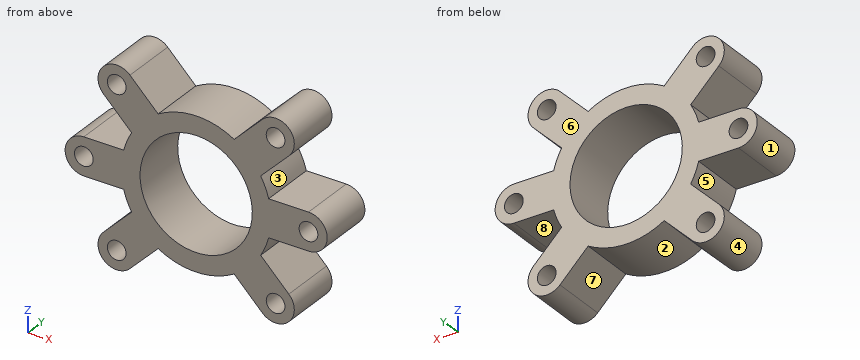
```python
from build123d import *

# Parameters (mm, degrees)
SKETCH2_R           = 30
SKETCH2_R_2         = 5
BOSS_EXTRUDE1_DEPTH = 15


with BuildPart() as part:
    # Sketch2 → Boss-Extrude1 (new, symmetric)
    with BuildSketch(Plane(origin=(0, 0, 0), x_dir=(1, 0, 0), z_dir=(0, 1, 0))):
        with BuildLine():
            Line((38.729833462, 10), (60, 10))
            ThreePointArc((60, 10), (70, 0), (60, -10))
            Line((60, -10), (38.729833462, -10))
            ThreePointArc((38.729833462, -10), (36.9551813, -15.307337295), (34.457195687, -20.315060063))
            Line((34.457195687, -20.315060063), (49.497474683, -35.355339059))
            ThreePointArc((49.497474683, -35.355339059), (49.497474683, -49.497474683), (35.355339059, -49.497474683))
            Line((35.355339059, -49.497474683), (20.315060063, -34.457195687))
            ThreePointArc((20.315060063, -34.457195687), (0, -40), (-20.315060063, -34.457195687))
            Line((-20.315060063, -34.457195687), (-35.355339059, -49.497474683))
            ThreePointArc((-35.355339059, -49.497474683), (-49.497474683, -49.497474683), (-49.497474683, -35.355339059))
            Line((-49.497474683, -35.355339059), (-34.457195687, -20.315060063))
            ThreePointArc((-34.457195687, -20.315060063), (-36.9551813, -15.307337295), (-38.729833462, -10))
            Line((-38.729833462, -10), (-60, -10))
            ThreePointArc((-60, -10), (-70, 0), (-60, 10))
            Line((-60, 10), (-38.729833462, 10))
            ThreePointArc((-38.729833462, 10), (-36.9551813, 15.307337295), (-34.457195687, 20.315060063))
            Line((-34.457195687, 20.315060063), (-49.497474683, 35.355339059))
            ThreePointArc((-49.497474683, 35.355339059), (-49.497474683, 49.497474683), (-35.355339059, 49.497474683))
            Line((-35.355339059, 49.497474683), (-20.315060063, 34.457195687))
            ThreePointArc((-20.315060063, 34.457195687), (0, 40), (20.315060063, 34.457195687))
            Line((20.315060063, 34.457195687), (35.355339059, 49.497474683))
            ThreePointArc((35.355339059, 49.497474683), (49.497474683, 49.497474683), (49.497474683, 35.355339059))
            Line((49.497474683, 35.355339059), (34.457195687, 20.315060063))
            ThreePointArc((34.457195687, 20.315060063), (36.9551813, 15.307337295), (38.729833462, 10))
        make_face()
        with Locations(Location((0, 0, 0), (0, 0, 270))):
            Circle(SKETCH2_R, mode=Mode.SUBTRACT)
        with Locations(Location((60, 0, 0), (0, 0, 270))):
            Circle(SKETCH2_R_2, mode=Mode.SUBTRACT)
        with Locations(Location((42.426406871, -42.426406871, 0), (0, 0, 270))):
            Circle(SKETCH2_R_2, mode=Mode.SUBTRACT)
        with Locations(Location((-42.426406871, -42.426406871, 0), (0, 0, 270))):
            Circle(SKETCH2_R_2, mode=Mode.SUBTRACT)
        with Locations(Location((-60, 0, 0), (0, 0, 270))):
            Circle(SKETCH2_R_2, mode=Mode.SUBTRACT)
        with Locations(Location((-42.426406871, 42.426406871, 0), (0, 0, 270))):
            Circle(SKETCH2_R_2, mode=Mode.SUBTRACT)
        with Locations(Location((42.426406871, 42.426406871, 0), (0, 0, 270))):
            Circle(SKETCH2_R_2, mode=Mode.SUBTRACT)
    extrude(amount=BOSS_EXTRUDE1_DEPTH, both=True)


solid = part.part
```
Check sheet for the modelled part. Datum: model origin and axes. Units: mm. Face numbers are marked on the shaded views. A direction names the side the tool comes from. Round coordinates to 2 decimals unless told otherwise and drop trailing zeros. Loops run counter-clockwise (first coordinate to the right, second up) from the corner with the lowest first, then second, coordinate; pieces in that order, holes last. Notation, with made-up numbers: (28, 50.5) - (49, 50.5) arc R24 ccw to (49, 80.5) - close; hole circle Ø6 at (70, 71). An arc over 180 degrees is marked (long way). Answer as a JSON object with one key per item and string values. Group by question number.
Q1. Sectioned sample at D-D, the plane x = -14.5. Enter the section's corners in (y, z), plus the area to 3 significant figures.
Q2. Set-up check for the marked faces 5, 6, 7 and 8: record each of +Z, -Z, +X, -X, +Y, -Y from which the full face is reachable in a straight line by a thin tool's end or side.
Q3. Mould release check, pull along X, two halves, no side actions. Record for the marked faces 1, 2, 3 and 4: released by +X, released by -X, zero draft, split by the parting line, or undercut.
Q4. Sectioned sample at A-A, the plane z = 0. Enter the section's corners in (x, y).
Q5. Sectioned sample at C-C, the plane y = 5. Count the separate pieces of the cut face and the enclosed holes in it, plus the area to 3 significant figures.
Q6. Gauge pin test, flat ends, axial feed: P1, Ø10.5, axis at x = -50, y = 0.5, coming from the +Z side; P2, Ø5, axis at x = -50.5, y = -9, coming from the -Z side; P3, Ø4, axis at x = 20, y = 8.5, coming from the -Z side. Record the tip position at first contact, or that the pin passes through.
Q7. Scan lines: line 1 along X through (y, z) = (0.5, 0); line 2 along Z through (x, y) = (42.5, 1.75); line 3 along Z through (x, y) = (40, 5). Record each from-to range of solid material in increasing order. Write a range as [from, to].
Q8. Sectioned sample at B-B, the plane x = 0. Enter the section's corners in (y, z), plus the area to 3 significant figures.
Solution:
{
 "1": {"outline": "(-15, -37.28) - (15, -37.28) - (15, -26.26) - (-15, -26.26) - close; (-15, 26.26) - (15, 26.26) - (15, 37.28) - (-15, 37.28) - close", "area": "661 mm²"},
 "2": {"face 5": "-X, +Y, -Y", "face 6": "+Z, -Z, +X, -X, +Y", "face 7": "-Z, +Y, -Y", "face 8": "+X, +Y, -Y"},
 "3": {"face 1": "released by -X", "face 2": "undercut", "face 3": "released by +X", "face 4": "undercut"},
 "4": {"outline": "(-70, -15) - (-65, -15) - (-65, 15) - (-70, 15) - close; (-55, -15) - (-30, -15) - (-30, 15) - (-55, 15) - close; (30, -15) - (55, -15) - (55, 15) - (30, 15) - close; (65, -15) - (70, -15) - (70, 15) - (65, 15) - close"},
 "5": {"separate pieces": "1", "enclosed holes": "7", "area": "5,120 mm²"},
 "6": {"P1": "stops at z = 52.15", "P2": "stops at z = -50.73", "P3": "stops at z = -36.14"},
 "7": {"line 1": "x = [-70, -65], [-55, -30], [30, 55], [65, 70]", "line 2": "z = [-52.43, -47.43], [-37.43, -28.36], [-10, 10], [28.36, 37.43], [47.43, 52.43]", "line 3": "z = [-52.13, -46.8], [-38.05, -25.86], [-10, 10], [25.86, 38.05], [46.8, 52.13]"},
 "8": {"outline": "(-15, -40) - (15, -40) - (15, -30) - (-15, -30) - close; (-15, 30) - (15, 30) - (15, 40) - (-15, 40) - close", "area": "600 mm²"}
}
